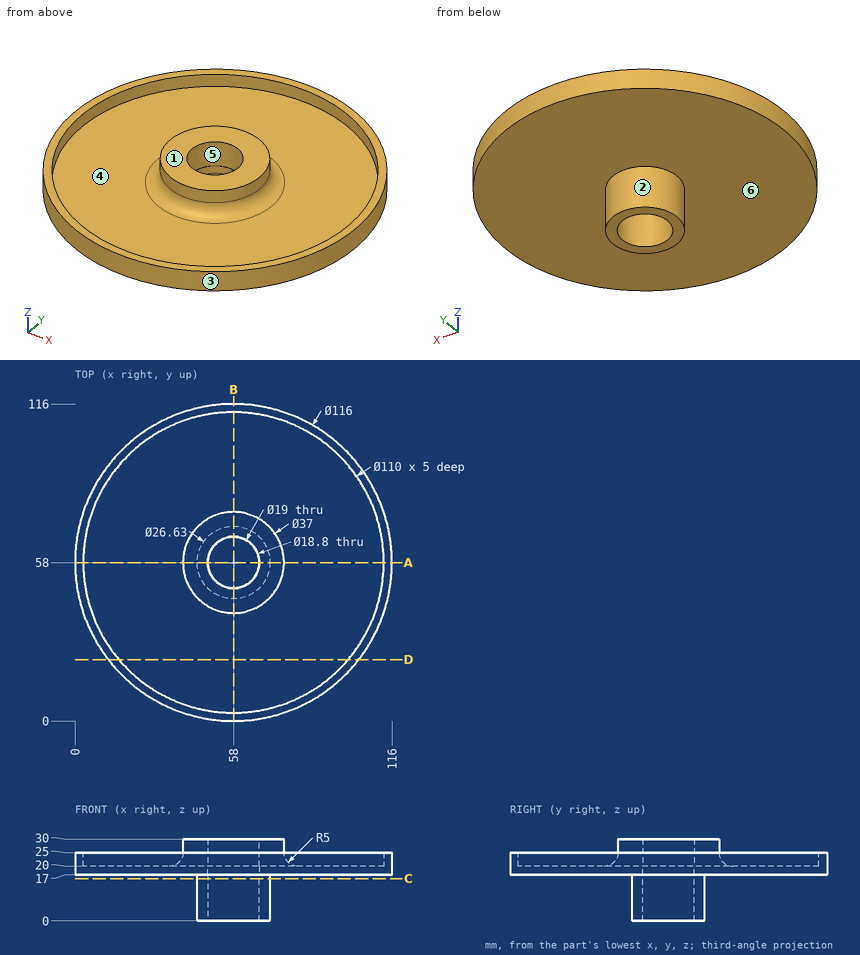
Could you check a few things on this drawing? It's one solid part, dimensions in mm from its lowest x, y, z. A direction names the side the tool comes from. Coordinates: 2 decimals unless noted, no trailing zeros. Order: outer loops, then holes, each group sorted by start corner. A loop starts at its lowest first (then second) coordinate and runs counter-clockwise, first axis right, second up. Notation, with made-up numbers: (14, 76) - (35, 76) arc R18 ccw to (35, 98) - close; hole circle Ø9 at (65, 52). An arc over 180 degrees is marked (long way). Answer as a JSON object with one key per item and string values. Group by question number.
Q1. We'd pull the mould along Y, two halves only. Please class the marked faces 3, 4, 5 and 6: +Y half, -Y half, draft (parallel to the pull), parting line (faces both ways), or undercut.
Q2. Imagine slicing it at A-A (y = 58). Please give me the cut outline in (x, z) (3 decimals).
Q3. Imagine slicing it at D-D (y = 22.5). Please give me the cut outline in (x, z), and give its area (3 significant figures).
Q4. I need wall thicknesses on line 1 (X direction, y = 58, z = 7) (3 decimals); line 2 (Y direction, x = 58, z = 18.3). Which ranges of each line are inside material? Lowest first, please. Write a range as from..to.
Q5. On a 3-axis mill with a long thin cutter (end or side, diameter ignored), from which of +Z, -Z, +X, -X, +Y, -Y can I reach the whole of each face in a straight line? I mean the marked faces 1 and 2. Say none if no direction works.
Q6. Imagine slicing it at C-C (z = 15.5). Please give me the cut outline in (x, y) (3 decimals).
Q7. Will these pins go through, and if not, where does the flat tip stop? P1, Ø10, axis at x = 26.5, z = 21.5, coming from the -Y side; P2, Ø4, axis at x = 51, y = 13, coming from the -Z side; P3, Ø12, axis at y = 67.5, z = 25.5, coming from the -X side; P4, Ø24.5, axis at x = 58, y = 58, coming from the +Z side.
Determined:
{
 "1": {"face 3": "parting line", "face 4": "undercut", "face 5": "undercut", "face 6": "draft"},
 "2": {"outline": "(0, 17) - (44.685, 17) - (44.685, 0) - (48.6, 0) - (48.6, 20) - (48.5, 20) - (48.5, 30) - (39.5, 30) - (39.5, 25) arc R5 cw to (34.5, 20) - (3, 20) - (3, 25) - (0, 25) - close; (67.4, 0) - (71.315, 0) - (71.315, 17) - (116, 17) - (116, 25) - (113, 25) - (113, 20) - (81.5, 20) arc R5 cw to (76.5, 25) - (76.5, 30) - (67.5, 30) - (67.5, 20) - (67.4, 20) - close"},
 "3": {"outline": "(12.13, 17) - (103.87, 17) - (103.87, 25) - (100.01, 25) - (100.01, 20) - (15.99, 20) - (15.99, 25) - (12.13, 25) - close", "area": "314 mm2"},
 "4": {"line 1": "x = 44.685..48.6, 67.4..71.315", "line 2": "y = 0..48.6, 67.4..116"},
 "5": {"face 1": "+Z, +X, -X, +Y, -Y", "face 2": "-Z"},
 "6": {"outline": "circle Ø26.63 at (58, 58); hole circle Ø18.8 at (58, 58)"},
 "7": {"P1": "stops at y = 6.41", "P2": "stops at z = 17", "P3": "stops at x = 0.11", "P4": "stops at z = 30"}
}
